Geometry: final body of the model. Coordinates: model frame, mm. Coordinates: 2 decimals unless noted, no trailing zeros. Loops run counter-clockwise (first coordinate to the right, second up) from the corner with the lowest first, then second, coordinate; pieces in that order, holes last. Notation, with made-up numbers: (66.25, 53.5) - (102.25, 53.5) arc R9 cw to (102.25, 68.5) - close; hole circle Ø5 at (-12, -38.5). An arc over 180 degrees is marked (long way). Answer in a Markdown table with one row per item.
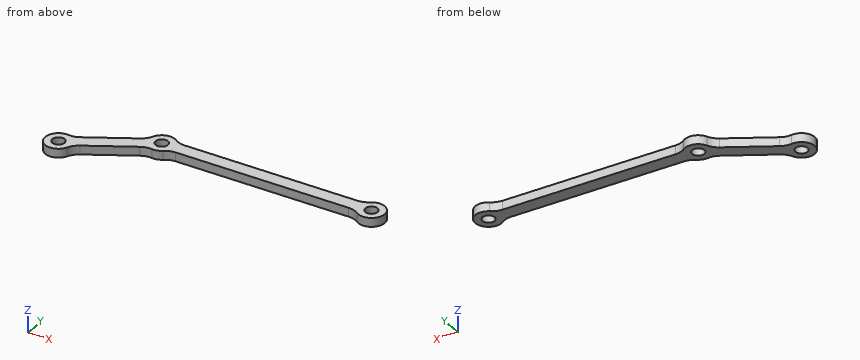
from build123d import *

# Parameters (mm, degrees)
SKETCH1_R          = 3.5
BASE_FLANGE1_DEPTH = 5
FILLET1_R          = 10


# Sheet-metal steps are written as plain solids
with BuildPart() as part:
    # Sketch1 → Base-Flange1 (new body)
    with BuildSketch(Plane.XY):
        with BuildLine():
            Line((-155.806954945, -25.29195723), (-123.494315244, -6.636246))
            ThreePointArc((-123.494315244, -6.636246), (-118.058857162, -7.244443697), (-113.65571123, -4))
            Line((-113.65571123, -4), (-6.34428877, -4))
            ThreePointArc((-6.34428877, -4), (7.5, 0), (-6.34428877, 4))
            Line((-6.34428877, 4), (-113.65571123, 4))
            ThreePointArc((-113.65571123, 4), (-121.941142838, 7.244443697), (-127.494315244, 0.29195723))
            Line((-127.494315244, 0.29195723), (-159.806954945, -18.363754))
            ThreePointArc((-159.806954945, -18.363754), (-169.796460718, -28.75), (-155.806954945, -25.29195723))
        make_face()
        Circle(SKETCH1_R, mode=Mode.SUBTRACT)
        with Locations((-120, 0)):
            Circle(SKETCH1_R, mode=Mode.SUBTRACT)
        with Locations((-163.301270189, -25)):
            Circle(SKETCH1_R, mode=Mode.SUBTRACT)
    extrude(amount=-BASE_FLANGE1_DEPTH)

    # Fillet1
    fillet1_edges = [part.edges().sort_by_distance(p)[0] for p in [
        (-159.806954945, -18.363754, -2.5),
        (-127.494315244, 0.29195723, -2.5),
        (-113.65571123, 4, -2.5),
        (-6.34428877, 4, -2.5),
        (-6.34428877, -4, -2.5),
        (-113.65571123, -4, -2.5),
        (-123.494315244, -6.636246, -2.5),
        (-155.806954945, -25.29195723, -2.5),
    ]]
    fillet(fillet1_edges, radius=FILLET1_R)


solid = part.part
(1) Cut plane B-B on z = -3.4. Output: boundary loops of the cut face in (x, y), then the cut area to 3 significant figures.
Verdict:
| item | result |
|---|---|
| outline | (-162.4, -17.55) arc R7.5 ccw (long way) to (-156.4, -27.95) arc R10 cw to (-152.21, -23.21) - (-127.09, -8.71) arc R10 cw to (-120.9, -7.45) arc R7.5 ccw to (-115.5, -6) arc R10 cw to (-109.5, -4) - (-10.5, -4) arc R10 cw to (-4.5, -6) arc R7.5 ccw (long way) to (-4.5, 6) arc R10 cw to (-10.5, 4) - (-109.5, 4) arc R10 cw to (-115.5, 6) arc R7.5 ccw to (-126.9, 2.95) arc R10 cw to (-131.09, -1.79) - (-156.21, -16.29) arc R10 cw to start; hole circle Ø7 at (-163.3, -25); hole circle Ø7 at (-120, 0); hole circle Ø7 at (0, 0) |
| area | 1,560 mm² |
(2) Cut plane D-D on x = -37.5. Output: boundary loops of the cut face in (y, z), then the cut area to 3 significant figures.
Verdict:
| item | result |
|---|---|
| outline | (-4, -5) - (4, -5) - (4, 0) - (-4, 0) - close |
| area | 40.0 mm² |
(3) Cut plane C-C on y = -25. Output: boundary loops of the cut face in (x, z), then the cut area to 3 significant figures.
Verdict:
| item | result |
|---|---|
| outline | (-170.8, -5) - (-166.8, -5) - (-166.8, 0) - (-170.8, 0) - close; (-159.8, -5) - (-154.47, -5) - (-154.47, 0) - (-159.8, 0) - close |
| area | 46.7 mm² |
(4) Cut plane A-A on x = 0. Output: boundary loops of the cut face in (y, z).
Verdict:
| item | result |
|---|---|
| outline | (-7.5, -5) - (-3.5, -5) - (-3.5, 0) - (-7.5, 0) - close; (3.5, -5) - (7.5, -5) - (7.5, 0) - (3.5, 0) - close |
(5) First-contact query: pin 1 Ø3 at (x, z) = (-103, -1.5) entering from -Y; pin 2 Ø2 at (y, z) = (-25.5, -2) entering from +X; pin 3 Ø11 at (x, y) = (-120, 0) entering from +Z; pin 4 Ø1 at (y, z) = (-14, -2) entering from +X. Flat tips, straight axial feed; report the tip coordinate or a pass-through.
Verdict:
| item | result |
|---|---|
| pin 1 | stops at y = -4 |
| pin 2 | stops at x = -153.96 |
| pin 3 | stops at z = 0 |
| pin 4 | stops at x = -135.38 |
(6) Ray query, probe 1 along Y at (x, z) = (-120, -2.9); probe 2 along Y at (x, z) = (-11, -0.55); probe 3 along Y at (x, z) = (-117, -3.9). Return the intervals inside material, ascending.
Verdict:
| item | result |
|---|---|
| probe 1 | y = -7.5 to -3.5, 3.5 to 7.5 |
| probe 2 | y = -4 to 4 |
| probe 3 | y = -6.87 to -1.8, 1.8 to 6.87 |
